```python
from build123d import *

# Parameters (mm, degrees)
F1_DEPTH = 7.5


# Not quite as in the source:
# - ends of sketch curves that miss each other by under 0.0002 mm in the source are joined


with BuildPart() as f1:
    # F0 (on Top) → F1 (new body)
    with BuildSketch(Plane.XY):
        with BuildLine():
            ThreePointArc((4.0556630512, -37.2800428811), (27.913593144, -25.0415917583), (37.5, 0))
            ThreePointArc((37.5, 0), (-25.0415917583, 27.913593144), (-4.0556630512, -37.2800428811))
            ThreePointArc((-4.0556630512, -37.2800428811), (-2.0308116554, -37.4449703434), (0, -37.5))
            ThreePointArc((0, -37.5), (2.0308116554, -37.4449703434), (4.0556630512, -37.2800428811))
        make_face()
        with BuildLine():
            ThreePointArc((-28.4078604382, -13.2949914876), (-27.1628882386, 15.6825009444), (-2.6901296616, 31.2494245665))
            Line((-2.6901296616, 31.2494245665), (7.92e-08, 32.8025716965))
            Line((7.92e-08, 32.8025716965), (2.6901298478, 31.2494245505))
            ThreePointArc((2.6901298478, 31.2494245505), (23.109946567, 21.2059827173), (31.365001727, 0))
            ThreePointArc((31.365001727, 0), (30.6167921454, -6.8099465531), (28.407860359, -13.2949916568))
            Line((28.407860359, -13.2949916568), (28.407860359, -16.4012859168))
            Line((28.407860359, -16.4012859168), (25.7177305905, -17.9544330629))
            ThreePointArc((25.7177305905, -17.9544330629), (-9.34e-08, -31.365001727), (-25.7177306974, -17.9544329097))
            Line((-25.7177306974, -17.9544329097), (-28.4078604382, -16.4012857797))
            Line((-28.4078604382, -16.4012857797), (-28.4078604382, -13.2949914876))
        make_face(mode=Mode.SUBTRACT)
        with BuildLine():
            ThreePointArc((-11.0725523918, -0.9414030915), (-9.6237073053, 5.5562499901), (-4.7209972243, 10.059813192))
            Line((-4.7209972243, 10.059813192), (-1.0416995056, 18.7393003948))
            Line((-1.0416995056, 18.7393003948), (-6.3499999208, 21.8040490685))
            Line((-6.3499999208, 21.8040490685), (-6.3499999208, 29.1363974872))
            Line((-6.3499999208, 29.1363974872), (-2.6901296616, 31.2494245665))
            ThreePointArc((-2.6901296616, 31.2494245665), (-27.1628882386, 15.6825009444), (-28.4078604382, -13.2949914876))
            Line((-28.4078604382, -13.2949914876), (-28.4078604382, -9.068937361))
            Line((-28.4078604382, -9.068937361), (-22.0578604382, -5.4027631516))
            Line((-22.0578604382, -5.4027631516), (-16.7495600286, -8.467511822))
            Line((-16.7495600286, -8.467511822), (-11.0725523918, -0.9414030915))
        make_face()
        with BuildLine():
            Line((6.3500000792, 21.8040490685), (1.0416996696, 18.739300398))
            Line((1.0416996696, 18.739300398), (4.7209974611, 10.0598130809))
            ThreePointArc((4.7209974611, 10.0598130809), (9.6237072938, 5.5562500099), (11.0725524179, -0.941402785))
            Line((11.0725524179, -0.941402785), (16.7495599439, -8.4675119624))
            Line((16.7495599439, -8.4675119624), (22.057860359, -5.4027632888))
            Line((22.057860359, -5.4027632888), (28.407860359, -9.0689374981))
            Line((28.407860359, -9.0689374981), (28.407860359, -13.2949916568))
            ThreePointArc((28.407860359, -13.2949916568), (30.6167921454, -6.8099465531), (31.365001727, 0))
            ThreePointArc((31.365001727, 0), (23.109946567, 21.2059827173), (2.6901298478, 31.2494245505))
            Line((2.6901298478, 31.2494245505), (6.3500000792, 29.1363974872))
            Line((6.3500000792, 29.1363974872), (6.3500000792, 21.8040490685))
        make_face()
        with BuildLine():
            Line((-6.3515551695, -9.1184101234), (-15.7078604382, -10.2717884324))
            Line((-15.7078604382, -10.2717884324), (-15.7078604382, -16.4012857797))
            Line((-15.7078604382, -16.4012857797), (-22.0578604382, -20.067459989))
            Line((-22.0578604382, -20.067459989), (-25.7177306974, -17.9544329097))
            ThreePointArc((-25.7177306974, -17.9544329097), (-9.34e-08, -31.365001727), (25.7177305905, -17.9544330629))
            Line((25.7177305905, -17.9544330629), (22.057860359, -20.0674601262))
            Line((22.057860359, -20.0674601262), (15.707860359, -16.4012859168))
            Line((15.707860359, -16.4012859168), (15.707860359, -10.271788576))
            Line((15.707860359, -10.271788576), (6.3515549548, -9.118410273))
            ThreePointArc((6.3515549548, -9.118410273), (-1.15e-08, -11.1125), (-6.3515551695, -9.1184101234))
        make_face()
    extrude(amount=F1_DEPTH)


solid = f1.part
```
Design review of the part built by this model. Coordinates are the model's own, in mm. Coordinates: 2 decimals unless noted, no trailing zeros. Write each loop counter-clockwise with the first axis right and the second up, starting at its lowest first coordinate (ties: lowest second). Pieces come first, ordered by that corner, then holes. Notation, with made-up numbers: M -24,-20 L 35,-20 A30 cw 35,13 Z; hole C 3.25,32.25 d7. An arc over 180 degrees is marked long. Answer as a JSON object with one key per item and string values.
Item 1: Add section D-D, the plane x = -30. Give the boundary of the cut face in (y, z).
Outcome:
{"outline": "M -22.5,0 L 22.5,0 L 22.5,7.5 L -22.5,7.5 Z"}
Item 2: Add section B-B, the plane y = -14. Give the boundary of the cut face in (x, z).
Outcome:
{"outline": "M -34.79,0 L -28.41,0 L -28.41,7.5 L -34.79,7.5 Z; M -15.71,0 L 15.71,0 L 15.71,7.5 L -15.71,7.5 Z; M 28.41,0 L 34.79,0 L 34.79,7.5 L 28.41,7.5 Z"}
Item 3: Draft analysis for pull direction Y (two halves, no side actions). For faces 1 (the flat face through (-15.708, -13, 4)), 2 (the flat face through (8, 9, 0)), 3 (the flat face through (13.87, -4.65, 3.7)), state which applies: pulls with the +Y half, pulls with the -Y half, needs draft (parallel to the pull), parting line crosses it, or undercut.
Outcome:
{"face 1": "undercut", "face 2": "needs draft", "face 3": "undercut"}
Item 4: Add section C-C, the plane y = -2. Give the boundary of the cut face in (x, z).
Outcome:
{"outline": "M -37.45,0 L -11.87,0 L -11.87,7.5 L -37.45,7.5 Z; M 11.87,0 L 37.45,0 L 37.45,7.5 L 11.87,7.5 Z"}
Item 5: Wall thickness on probe 1 along Y at (x, z) = (5, 1.75); probe 2 along X at (y, z) = (-14.5, 5.75); probe 3 along Y at (x, z) = (2.5, 1): over which ranges is each line inside the solid? List them lowest first.
Outcome:
{"probe 1": "-37.17 to -9.92, 9.92 to 21.02, 29.92 to 37.17", "probe 2": "-34.58 to -28.41, -15.71 to 15.71, 28.41 to 34.58", "probe 3": "-37.42 to -10.83, 15.3 to 19.58, 31.36 to 37.42"}
Item 6: Insertion check: pin 1 Ø3 at (y, z) = (19.5, 5) entering from -X; pin 2 Ø3 at (x, z) = (-2.5, 1.5) entering from -Y; pin 3 Ø3.5 at (y, z) = (26, 5) entering from -X; pin 4 Ø8 at (x, y) = (-22, -2) entering from -Z. Each pin has a flat end and moves straight along its axis. Give the tip position at first contact, or say it passes through.
Outcome:
{"pin 1": "x = -32.9", "pin 2": "y = -37.49", "pin 3": "x = -28.6", "pin 4": "z = 0"}
Item 7: Add section A-A, the plane x = -19.5. Give the boundary of the cut face in (y, z).
Outcome:
{"outline": "M -32.03,0 L -18.59,0 L -18.59,7.5 L -32.03,7.5 Z; M -6.88,0 L 32.03,0 L 32.03,7.5 L -6.88,7.5 Z"}
